Autodesk Inventor part; units mm, degrees
ref_plane "YZ Plane" through (0, 0, 0) normal (1, 0, 0) x (0, 1, 0)
ref_plane "XZ Plane" through (0, 0, 0) normal (0, 1, 0) x (-1, 0, 0)
ref_plane "XY Plane" through (0, 0, 0) normal (0, 0, 1) x (1, 0, 0)
sketch "Sketch1" plane through (0, 0, 0) normal (0, 0, 1) x (1, 0, 0)
  line L0 (24, 7.65) -> (-24, 7.65)
  line L1 (-24, 7.65) -> (-24, -7.65)
  line L2 (-24, -7.65) -> (24, -7.65)
  line L3 (24, -7.65) -> (24, 7.65)
  line L4 (24, 7.65) -> (-24, -7.65) construction
  line L5 (-24, 7.65) -> (24, -7.65) construction
  line L6 (-22.5, -7.65) -> (-15.5, -7.65)
  line L7 (-15.5, -7.65) -> (-15.5, -10.45)
  line L8 (-15.5, -10.45) -> (-22.5, -10.45)
  line L9 (-22.5, -10.45) -> (-22.5, -7.65)
  line L10 (22.5, -7.65) -> (13.5, -7.65)
  line L11 (13.5, -7.65) -> (13.5, -10.45)
  line L12 (13.5, -10.45) -> (22.5, -10.45)
  line L13 (22.5, -10.45) -> (22.5, -7.65)
  line L14 (24, -5.95) -> (27, -5.95)
  line L15 (27, -5.95) -> (27, 4.05)
  line L16 (27, 4.05) -> (24, 4.05)
  line L17 (24, 4.05) -> (24, -5.95)
  line L18 (-24, -5.95) -> (-27, -5.95)
  line L19 (-27, -5.95) -> (-27, 4.05)
  line L20 (-27, 4.05) -> (-24, 4.05)
  line L21 (-24, 4.05) -> (-24, -5.95)
  line L22 (-12.5, -7.65) -> (12.5, -7.65)
  line L23 (12.5, -7.65) -> (12.5, -4.85)
  line L24 (12.5, -4.85) -> (-12.5, -4.85)
  line L25 (-12.5, -4.85) -> (-12.5, -7.65)
  circle A0 centre (15, 19.55) radius 1.75
  arc A1 (19.768, 21.0552) -> (12.9654, 24.1173) centre (15, 19.55) ccw
  line L26 (-24, 7.65) -> (12.9654, 24.1173)
  line L27 (24, 7.65) -> (19.768, 21.0552)
  point P0 (0, 0)
  point P1 (-25.5, -5.95)
  point P2 (25.5, -5.95)
  point P3 (25.5, 4.05)
  point P4 (-25.5, 4.05)
  point P5 (0, -4.85)
  point P6 (0, 0)
  dimension "d0" = 48
  dimension "d1" = 15.3
  dimension "d2" = 3.5
  dimension "d3" = 30
  dimension "d4" = 2.8
  dimension "d5" = 12
  dimension "d6" = 3
  dimension "d7" = 4.5
  dimension "d8" = 10
  dimension "d9" = 25
  dimension "d10" = 7
  dimension "d11" = 9
  dimension "d12" = 4.5
  dimension "d13" = 4.5
  dimension "d14" = 10
extrude "Extrusion1" add sketch "Sketch1" along normal mid plane 2.8 contours L3 L2 L23 L24 L25 L1 L0 | L0 L26 A1 L27 | L16 L15 L14 L3 | L1 L18 L19 L20 | L13 L12 L11 L2 | L2 L7 L8 L9
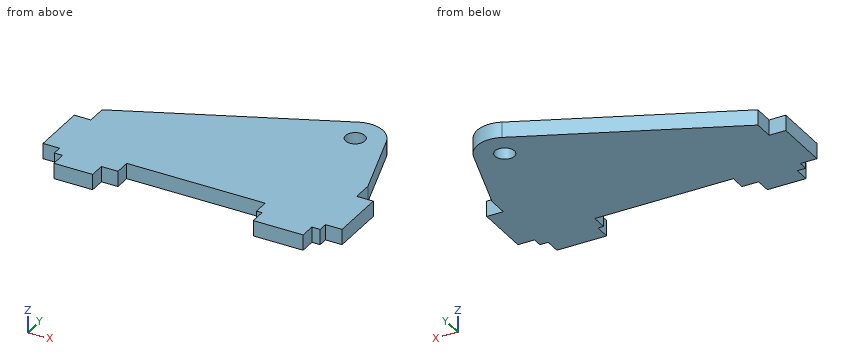
Input: part model. Units: mm. Frame: model coordinates. Round coordinates to 2 decimals unless told otherwise and drop trailing zeros. Order: outer loops, then holes, each group sorted by start corner. A loop starts at its lowest first (then second) coordinate and runs counter-clockwise, first axis right, second up.
1. Material intervals for line 1 (Y direction, x = 15, z = 0.05); line 2 (Y direction, x = 16, z = 0.55); line 3 (Y direction, x = -25, z = 0.95), sorted ascending.
The answers:
line 1: y = -10.45 to 17.8, 21.3 to 24.55
line 2: y = -10.45 to 18.11, 20.99 to 24.45
line 3: y = -5.95 to 4.05
2. Cut plane C-C, the plane z = 0.4. Output: boundary loops of the cut face in (x, y), then the cut area to 3 significant figures.
The answers:
outline: (-27, -5.95) - (-24, -5.95) - (-24, -7.65) - (-22.5, -7.65) - (-22.5, -10.45) - (-15.5, -10.45) - (-15.5, -7.65) - (-12.5, -7.65) - (-12.5, -4.85) - (12.5, -4.85) - (12.5, -7.65) - (13.5, -7.65) - (13.5, -10.45) - (22.5, -10.45) - (22.5, -7.65) - (24, -7.65) - (24, -5.95) - (27, -5.95) - (27, 4.05) - (24, 4.05) - (24, 7.65) - (19.77, 21.06) arc R5 ccw to (12.97, 24.12) - (-24, 7.65) - (-24, 4.05) - (-27, 4.05) - close; hole circle Ø3.5 at (15, 19.55)
area: 1,200 mm2
3. Cut plane D-D, the plane y = 12.5. Output: boundary loops of the cut face in (x, z).
The answers:
outline: (-13.11, -1.4) - (22.47, -1.4) - (22.47, 1.4) - (-13.11, 1.4) - close
4. Cut plane B-B, the plane x = 15. Output: boundary loops of the cut face in (y, z).
The answers:
outline: (-10.45, -1.4) - (17.8, -1.4) - (17.8, 1.4) - (-10.45, 1.4) - close; (21.3, -1.4) - (24.55, -1.4) - (24.55, 1.4) - (21.3, 1.4) - close
5. Cut plane A-A, the plane y = -7. Output: boundary loops of the cut face in (x, z), then the cut area to 3 significant figures.
The answers:
outline: (-24, -1.4) - (-12.5, -1.4) - (-12.5, 1.4) - (-24, 1.4) - close; (12.5, -1.4) - (24, -1.4) - (24, 1.4) - (12.5, 1.4) - close
area: 64.4 mm2
6. Pin query (flat end, axial travel): P1, Ø3, axis at x = 15, y = 19.55, coming from the +Z side; P2, Ø0.8, axis at x = 13, z = 0.5, coming from the -Y side; P3, Ø1.4, axis at x = 25, z = 0, coming from the -Y side; P4, Ø0.8, axis at y = 5.5, z = 0, coming from the -X side. Return the tip coordinate at first contact, or that it passes through.
The answers:
P1: passes through
P2: stops at y = -7.65
P3: stops at y = -5.95
P4: stops at x = -24
